For this review, take the finished solid that the model builds, in its own axes (mm). A direction names the side the tool comes from. Give positions to 0.01 mm unless a question says otherwise; leave off trailing zeros. Loops run counter-clockwise (first coordinate to the right, second up) from the corner with the lowest first, then second, coordinate; pieces in that order, holes last. Notation, with made-up numbers: (84, 42.5) - (103, 42.5) arc R14 cw to (103, 49.5) - close; hole circle Ø6 at (20.25, 45). An arc over 180 degrees is marked (long way). Put each result on its own line as item: value.
from build123d import *

# Parameters (mm, degrees)
SKETCH1_W           = 25
SKETCH1_H           = 25
SKETCH1_W_2         = 23
SKETCH1_H_2         = 23
BOSS_EXTRUDE1_DEPTH = 1200
CUT_EXTRUDE1_DEPTH  = 1201.325476694


with BuildPart() as part:
    # Sketch1 → Boss-Extrude1 (new body)
    with BuildSketch(Plane(origin=(0, 0, 0), x_dir=(1, 0, 0), z_dir=(0, 1, 0))):
        Rectangle(SKETCH1_W, SKETCH1_H)
        Rectangle(SKETCH1_W_2, SKETCH1_H_2, mode=Mode.SUBTRACT)
    extrude(amount=BOSS_EXTRUDE1_DEPTH)

    # Sketch2 → Cut-Extrude1 (cut, through all)
    with BuildSketch(Plane(origin=(12.5, 0, 0), x_dir=(0, 0, -1), z_dir=(1, 0, 0))):
        Polygon((12.5, 0), (-12.5, 5.313914042), (-12.5, 0), align=None)
        Polygon((12.5, 1200), (-12.5, 1200), (-12.5, 986.760885112), (12.5, 981.44697107), align=None)
    extrude(amount=-CUT_EXTRUDE1_DEPTH, mode=Mode.SUBTRACT)


solid = part.part
1) Insertion check: pin 1 Ø12 at (x, z) = (8, -2) entering from -Y. The pin has a flat end and moves straight along its axis. Give the tip position at first contact, or say it passes through.
Geometry check:
pin 1: stops at y = 1.2
2) Wall thickness on line 1 (X direction, y = 665, z = 5): over which ranges is the line inside the solid? List them lowest first.
Geometry check:
line 1: x = -12.5 to -11.5, 11.5 to 12.5
3) Take a section at B-B on y = 534.5. State the section outline as (x, z) points.
Geometry check:
outline: (-12.5, -12.5) - (12.5, -12.5) - (12.5, 12.5) - (-12.5, 12.5) - close; hole (-11.5, -11.5) - (11.5, -11.5) - (11.5, 11.5) - (-11.5, 11.5) - close
4) Take a section at C-C on z = 6. State the section outline as (x, y) points.
Geometry check:
outline: (-12.5, 3.93) - (-11.5, 3.93) - (-11.5, 985.38) - (-12.5, 985.38) - close; (11.5, 3.93) - (12.5, 3.93) - (12.5, 985.38) - (11.5, 985.38) - close
5) Draft analysis for pull direction X (two halves, no side actions). For faces 3 (the face through (-12.5, 486, 0)), 4 (the face through (0, 489, 11.5)), 5 (the face through (12.5, 486, 0)), state which applies: pulls with the +X half, pulls with the -X half, needs draft (parallel to the pull), parting line crosses it, or undercut.
Geometry check:
face 3: pulls with the -X half
face 4: undercut
face 5: pulls with the +X half
6) Take a section at A-A on x = -6.25. State the section outline as (y, z) points, and give its area (3 significant figures).
Geometry check:
outline: (0, -12.5) - (981.45, -12.5) - (981.66, -11.5) - (0.21, -11.5) - close; (5.1, 11.5) - (986.55, 11.5) - (986.76, 12.5) - (5.31, 12.5) - close
area: 1,960 mm²
7) For faces 1 (the face through (-11.5, 486, 0)), 2 (the face through (-11.98, 2.45, -0.98)), list the 3-axis set-ups (+Z, -Z, +X, -X, +Y, -Y) from which the entire face can be reached by the end or side of a thin tool; tool diameter is ignored.
Geometry check:
face 1: +Y, -Y
face 2: +Z, +X, -X, -Y
